Part model, mm, in its own coordinate system. Face numbers are marked on the shaded views. A direction names the side the tool comes from. Give positions to 0.01 mm unless a question says otherwise; leave off trailing zeros. Order: outer loops, then holes, each group sorted by start corner. A loop starts at its lowest first (then second) coordinate and runs counter-clockwise, first axis right, second up. Notation, with made-up numbers: M 89.25,70.5 L 115.25,70.5 A5 ccw 115.25,77.5 Z; hole C 57.25,48.25 d11. An arc over 180 degrees is marked long. Answer as a JSON object with one key per item and string values.
from build123d import *

# Parameters (mm, degrees)
FILLET1_R                       = 10.16
F_11_16_0_6875_DIAMETER_HOLE1_D = 17.4625
CIRPATTERN1_COUNT               = 8


with BuildPart() as part:
    # Sketch1 → Revolve1 (revolve)
    with BuildSketch(Plane.XY):
        Polygon((50.8, -152.4), (66.675, -152.4), (66.675, 0), (127, 0), (127, 15.875), (69.85, 15.875), (69.85, 10.795), (60.325, 10.795), (60.325, 15.875), (50.8, 15.875), align=None)
    revolve(axis=Axis((0, 66.332099957, 0), (0, -1, 0)))

    # Fillet1
    fillet1_edges = [part.edges().sort_by_distance(p)[0] for p in [
        (-66.675, 0, 0),
    ]]
    fillet(fillet1_edges, radius=FILLET1_R)

    # 11_16 _0.6875_ Diameter Hole1 (through all)
    with Locations(Plane(origin=(0, 15.875, 0), x_dir=(-1, 0, 0), z_dir=(0, 1, 0))):
        with Locations((0, -101.6)):
            f_11_16_0_6875_diameter_hole1 = Hole(F_11_16_0_6875_DIAMETER_HOLE1_D / 2)

    # CirPattern1: 11_16 _0.6875_ Diameter Hole1 ×8 about axis
    cirpattern1_axis = Axis((0, 0, 0), (0, 1, 0))
    for i in range(1, CIRPATTERN1_COUNT):
        add(f_11_16_0_6875_diameter_hole1.rotate(cirpattern1_axis, i * 360 / CIRPATTERN1_COUNT), mode=Mode.SUBTRACT)


solid = part.part
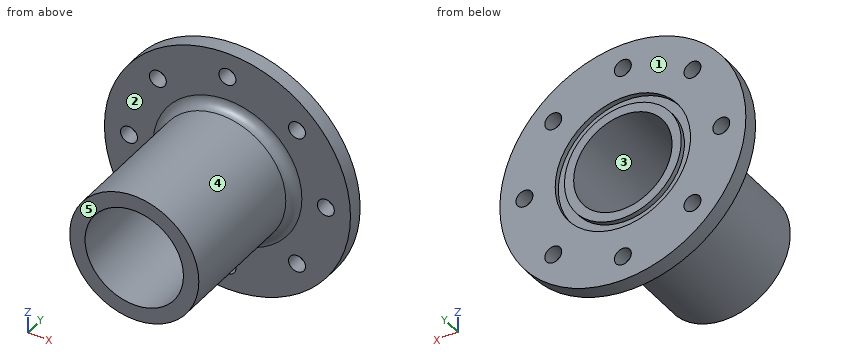
1. Cut at B-B on z = -101.6. Give the cut face in (x, y) (3 decimals).
Worked answers:
{"outline": "M -76.2,0 L -8.731,0 L -8.731,15.875 L -76.2,15.875 Z; M 8.731,0 L 76.2,0 L 76.2,15.875 L 8.731,15.875 Z"}
2. Two-plate mould, pull along X, no slides. Class the marked faces 3, 4 and 5: +X half, -X half, draft (parallel to the pull), parting line (faces both ways), or undercut.
Worked answers:
{"face 3": "undercut", "face 4": "parting line", "face 5": "draft"}
3. Which spindle directions (+Z, -Z, +X, -X, +Y, -Y) get a long thin tool onto all of the face, cutting with end or side? Do the marked faces 1 and 2. Say none if no direction does.
Worked answers:
{"face 1": "+Z, -Z, +X, -X, +Y", "face 2": "-Y"}
4. Probe line 1 along Z through (x, y) = (0, 14) (3 decimals); line 2 along Y through (x, z) = (0, 83) (3 decimals); line 3 along Z through (x, y) = (-46, -142). List the from-to ranges inside material, lowest first.
Worked answers:
{"line 1": "z = -127 to -110.331, -92.869 to -69.85, -60.325 to -50.8, 50.8 to 60.325, 69.85 to 92.869, 110.331 to 127", "line 2": "y = 0 to 15.875", "line 3": "z = -48.27 to -21.56, 21.56 to 48.27"}
5. Cut at D-D on x = -101.6. Give the cut face in (y, z) (3 decimals).
Worked answers:
{"outline": "M 0,-76.2 L 15.875,-76.2 L 15.875,-8.731 L 0,-8.731 Z; M 0,8.731 L 15.875,8.731 L 15.875,76.2 L 0,76.2 Z"}
6. Pin check, flat tips, straight feed: P1, Ø8, axis at y = -75.5, z = -54.5, coming from the +X side; P2, Ø10, axis at y = -44.5, z = 25.5, coming from the -X side; P3, Ø2, axis at x = -59.5, y = -77.5, coming from the +Z side; P4, Ø20, axis at x = 0, z = 101.6, coming from the +Y side (3 decimals). Stop position of each tip, or through.
Worked answers:
{"P1": "stops at x = 43.54", "P2": "stops at x = -63.45", "P3": "stops at z = 31.99", "P4": "stops at y = 15.875"}
7. Cut at A-A on x = 0. State how many separate pieces and enclosed holes the cut face has, plus the area to 3 significant figures.
Worked answers:
{"separate pieces": "4", "enclosed holes": "0", "area": "6,650 mm^2"}
